Work out the finished part from the listing and answer in its coordinate system (mm). A direction names the side the tool comes from. Give positions to 0.01 mm unless a question says otherwise; leave off trailing zeros. Write each loop counter-clockwise with the first axis right and the second up, starting at its lowest first coordinate (ties: lowest second). Pieces come first, ordered by that corner, then holes.
1) Find section C-C (y = 6). Determine the outline of the cut face in (x, z), plus the area to 3 significant figures.
2) Straight lines are drawn through the part: probe 1 along Y at (x, z) = (-2.5, 0.4); probe 2 along Y at (x, z) = (0.5, 0.9); probe 3 along X at (y, z) = (20, 0.7). For each, find the intervals that lie inside material, in ascending order.
3) Find section B-B (z = 2.4). Determine the outline of the cut face in (x, y).
4) Find section D-D (x = 9). Determine the outline of the cut face in (y, z).
5) Determine the mould class of faces 4 (the face through (6.81, -33.45, 1.97)), 5 (the face through (-0.328, 0.166, 1.972)), 6 (the face through (-3.803, 24, 2)), 7 (the face through (0, 14.51, 2)) for opening direction Y: pulls with the +Y half, pulls with the -Y half, needs draft (parallel to the pull), parting line crosses it, or undercut.
6) Find section A-A (x = -2.25). Determine the outline of the cut face in (y, z).
7) Given pin 1 Ø1.5 at (y, z) = (11, 3) entering from +X; pin 2 Ø1.2 at (x, z) = (2, 1.5) entering from -Y; pin 3 Ø0.8 at (x, z) = (2, 1) entering from +Y, each flat-ended and moving along its own axis, determine where each tip first touches the part or whether it passes through.
8) A tool of negligible diameter and unlimited length cuts with its end or side. For faces 1 (the face through (2, 20.11, 2)), 2 (the face through (-7.803, 7, 2)), 3 (the face through (3.797, 24, 2)), from which of +Z, -Z, +X, -X, +Y, -Y can it reach the whole face along a straight path? Write none if from no direction.
```python
from build123d import *

# Parameters (mm, degrees)
SKETCH_1_R      = 4.25
SKETCH_1_R_2    = 3.8
SKETCH_1_R_3    = 1.5
EXTRUDE_1_DEPTH = 4


with BuildPart() as part:
    # 草图1 → 凸台-拉伸1 (new body)
    with BuildSketch(Plane.XY):
        with BuildLine():
            Line((1.497207067, 22.610079684), (3.797207067, 22.610079684))
            Line((3.797207067, 22.610079684), (3.797207067, 24.610079684))
            Line((3.797207067, 24.610079684), (7.797207067, 24.610079684))
            Line((7.797207067, 24.610079684), (7.797207067, -9.232125177))
            ThreePointArc((7.797207067, -9.232125177), (9.997207067, -15.489920316), (7.797207067, -21.747715455))
            Line((7.797207067, -21.747715455), (5.797207067, -45.489920316))
            ThreePointArc((5.797207067, -45.489920316), (-0.002792933, -51.289920316), (-5.802792933, -45.489920316))
            Line((-5.802792933, -45.489920316), (-7.802792933, -21.747715455))
            ThreePointArc((-7.802792933, -21.747715455), (-10.002792933, -15.489920316), (-7.802792933, -9.232125177))
            Line((-7.802792933, -9.232125177), (-7.802792933, 24.610079684))
            Line((-7.802792933, 24.610079684), (-3.802792933, 24.610079684))
            Line((-3.802792933, 24.610079684), (-3.802792933, 22.610079684))
            Line((-3.802792933, 22.610079684), (-1.502792933, 22.610079684))
            Line((-1.502792933, 22.610079684), (-1.502792933, 20.110079684))
            Line((-1.502792933, 20.110079684), (-3.002792933, 20.110079684))
            Line((-3.002792933, 20.110079684), (-3.002792933, 17.510079684))
            Line((-3.002792933, 17.510079684), (-1.502792933, 17.510079684))
            Line((-1.502792933, 17.510079684), (-1.502792933, 14.510079684))
            Line((-1.502792933, 14.510079684), (1.497207067, 14.510079684))
            Line((1.497207067, 14.510079684), (1.497207067, 17.510079684))
            Line((1.497207067, 17.510079684), (2.997207067, 17.510079684))
            Line((2.997207067, 17.510079684), (2.997207067, 20.110079684))
            Line((2.997207067, 20.110079684), (1.497207067, 20.110079684))
            Line((1.497207067, 20.110079684), (1.497207067, 22.610079684))
        make_face()
        with Locations((-0.002792933, -15.489920316)):
            Circle(SKETCH_1_R, mode=Mode.SUBTRACT)
        with Locations((-0.002792933, -45.489920316)):
            Circle(SKETCH_1_R_2, mode=Mode.SUBTRACT)
        with Locations((-0.002792933, 1.630079684)):
            Circle(SKETCH_1_R_3, mode=Mode.SUBTRACT)
    extrude(amount=EXTRUDE_1_DEPTH)


solid = part.part
```
Results:
1. outline: (-7.8, 0) - (7.8, 0) - (7.8, 4) - (-7.8, 4) - close
1. area: 62.4 mm2
2. probe 1: y = -50.72 to -48.35, -42.63 to -18.93, -12.05 to 17.51, 20.11 to 22.61
2. probe 2: y = -51.27 to -49.26, -41.72 to -19.71, -11.27 to 0.22, 3.04 to 14.51
2. probe 3: x = -7.8 to -3, 3 to 7.8
3. outline: (-7.8, -21.75) - (-5.8, -45.49) arc R5.8 ccw to (5.8, -45.49) - (7.8, -21.75) arc R10 ccw to (7.8, -9.23) - (7.8, 24.61) - (3.8, 24.61) - (3.8, 22.61) - (1.5, 22.61) - (1.5, 20.11) - (3, 20.11) - (3, 17.51) - (1.5, 17.51) - (1.5, 14.51) - (-1.5, 14.51) - (-1.5, 17.51) - (-3, 17.51) - (-3, 20.11) - (-1.5, 20.11) - (-1.5, 22.61) - (-3.8, 22.61) - (-3.8, 24.61) - (-7.8, 24.61) - (-7.8, -9.23) arc R10 ccw to start; hole circle Ø8.5 at (0, -15.49); hole circle Ø7.6 at (0, -45.49); hole circle Ø3 at (0, 1.63)
4. outline: (-19.84, 0) - (-11.14, 0) - (-11.14, 4) - (-19.84, 4) - close
5. face 4: pulls with the -Y half
5. face 5: undercut
5. face 6: needs draft
5. face 7: pulls with the +Y half
6. outline: (-50.84, 0) - (-48.55, 0) - (-48.55, 4) - (-50.84, 4) - close; (-42.43, 0) - (-19.1, 0) - (-19.1, 4) - (-42.43, 4) - close; (-11.88, 0) - (17.51, 0) - (17.51, 4) - (-11.88, 4) - close; (20.11, 0) - (22.61, 0) - (22.61, 4) - (20.11, 4) - close
7. pin 1: stops at x = 7.8
7. pin 2: stops at y = -51.12
7. pin 3: stops at y = 22.61
8. face 1: +Z, -Z
8. face 2: +Z, -Z, -X, +Y
8. face 3: +Z, -Z, +Y
